```python
from build123d import *

# Parameters (mm, degrees)
PAD003_DEPTH            = 50.8
BODY003_PLACEMENT_ANGLE = 15


with BuildPart() as part:
    # Sketch003 → Pad003 (new body)
    with BuildSketch(Plane.XZ):
        with BuildLine():
            Line((-130.379928, 312.132536), (-130.379928, 159.732536))
            Line((-130.379928, 159.732536), (22.020072, 159.732536))
            Line((22.020072, 261.332536), (22.020072, 159.732536))
            Line((72.820072, 261.332536), (22.020072, 261.332536))
            Line((72.820072, 159.732536), (72.820072, 261.332536))
            Line((72.820072, 159.732536), (1190.420072, 159.732536))
            Line((1190.420072, 261.332536), (1190.420072, 159.732536))
            Line((1241.220072, 261.332536), (1190.420072, 261.332536))
            Line((1241.220072, 159.732536), (1241.220072, 261.332536))
            Line((1241.220072, 159.732536), (1393.620072, 159.732536))
            Line((1393.620072, 159.732536), (1393.620072, 312.132536))
            ThreePointArc((1393.620072, 312.132536), (1304.346219, 527.658683), (1088.820072, 616.932536))
            Line((1088.820072, 616.932536), (174.420072, 616.932536))
            ThreePointArc((174.420072, 616.932536), (-41.106075, 527.658683), (-130.379928, 312.132536))
        make_face()
    extrude(amount=PAD003_DEPTH)


with BuildPart() as part_1:
    # Body003 placement: moved
    add(part.part.moved(Location((0, 183.716529, -79.469557))).rotate(Axis((0, 183.716529, -79.469557), (-1, 0, 0)), BODY003_PLACEMENT_ANGLE))


solid = part_1.part
```
The listing builds one solid part. Answer for the finished solid, in the listing's coordinates (mm). A direction names the side the tool comes from. Coordinates: 2 decimals unless noted, no trailing zeros. Write each loop counter-clockwise with the first axis right and the second up, starting at its lowest first coordinate (ties: lowest second). Pieces come first, ordered by that corner, then holes. Notation, with made-up numbers: (-31.5, 16.25) - (-0.5, 16.25) arc R12 ccw to (-0.5, 37.25) - close; hole circle Ø5 at (74, -30.75). An arc over 180 degrees is marked (long way). Return JSON: item names as keys, results as strings. Group by question number.
1. A cutting plane is placed at A-A, the plane z = 144. Determine the outline of the cut face in (x, y), plus the area to 3 significant figures.
2. Which of the six approach directions +Z, -Z, +X, -X, +Y, -Y give full straight-line access (tool end or side, diameter ignored) to faces 1 (the flat face through (623.8, 200.87, 81.3)), 2 (the flat face through (47.78, 227.16, 179.44))?
3. A cutting plane is placed at C-C, the plane x = 1213.5. Determine the outline of the cut face in (y, z).
4. Straight lines are drawn through the part: L1, parallel to X at y = 204.5, z = 168; L2, parallel to X at y = 221, z = 240; L3, parallel to Y at x = 982.5, z = 472.5. For each, find the intervals that lie inside material, in ascending order.
5. A cutting plane is placed at B-B, the plane x = 997. Determine the outline of the cut face in (y, z).
6. Given pin 1 (5 mm diameter, centred on y = 289.5, z = 405.5, fed in from +X); pin 2 (1 mm diameter, centred on x = 1230.5, z = 379, fed in from +Y); pin 3 (6 mm diameter, centred on x = 202.5, z = 227, fed in from +Y), each flat-ended and moving along its own axis, determine where each tip first touches the part or whether it passes through.
7. Determine the mould class of faces 3 (the flat face through (620.952, 285.053, 298.722)), 4 (the flat face through (1393.62, 220, 154)), 5 (the flat face through (1216.18, 227.16, 179.44)) for opening direction X: released by +X, released by -X, zero draft, split by the parting line, or undercut.
Ans:
{
 "1": {"outline": "(-130.38, 191) - (22.02, 191) - (22.02, 243.6) - (-130.38, 243.6) - close; (72.82, 191) - (1190.42, 191) - (1190.42, 243.6) - (72.82, 243.6) - close; (1241.22, 191) - (1393.62, 191) - (1393.62, 243.6) - (1241.22, 243.6) - close", "area": "74,800 mm²"},
 "2": {"face 1": "-Z, +X, -X, -Y", "face 2": "-Z, -Y"},
 "3": {"outline": "(202.29, 186.11) - (251.35, 172.96) - (336.49, 490.68) - (287.42, 503.83) - close"},
 "4": {"L1": "-130.38 to 22.02, 72.82 to 1190.42, 1241.22 to 1393.62", "L2": "-130.32 to 1393.56", "L3": "279.02 to 331.62"},
 "5": {"outline": "(175.99, 87.97) - (225.06, 74.82) - (343.39, 516.44) - (294.32, 529.59) - close"},
 "6": {"pin 1": "x = 1333.92", "pin 2": "y = 306.7", "pin 3": "y = 266.64"},
 "7": {"face 3": "zero draft", "face 4": "released by +X", "face 5": "undercut"}
}
